Design review of the part built by this model. Coordinates are the model's own, in mm. A direction names the side the tool comes from. Coordinates: 2 decimals unless noted, no trailing zeros. Write each loop counter-clockwise with the first axis right and the second up, starting at its lowest first coordinate (ties: lowest second). Pieces come first, ordered by that corner, then holes. Notation, with made-up numbers: (54.5, 48.25) -> (66.5, 48.25) arc R12 cw to (66.5, 55.25) -> close; hole circle Ø11 at (42.5, 39). An arc over 180 degrees is marked (long way). Answer in a Markdown table with one row per item. Add a question column.
Item 1: Take a section at D-D, the plane x = -70.5. Write out the cut boundary in (y, z), and give its area (3 significant figures).
Item 2: Take a section at B-B, the plane z = -40. Write out the cut boundary in (x, y), and give its area (3 significant figures).
Item 3: For faces 1 (the face through (-39.44, 22.6, -15.77)), 2 (the face through (-40, -160, -40)), 3 (the face through (-32.68, -78.88, -41.63)), list the 3-axis set-ups (+Z, -Z, +X, -X, +Y, -Y) from which the entire face can be reached by the end or side of a thin tool; tool diameter is ignored.
Item 4: To check wall thickness, follow line 1 (Y direction, x = -27, z = -31); line 2 (Y direction, x = -51, z = -12.5); line 3 (Y direction, x = -41, z = -25). State the ranges of each line that lie inside material, in increasing order.
Item 5: Take a section at C-C, the plane x = -40. Write out the cut boundary in (y, z), and give its area (3 significant figures).
Item 6: Clearance check with flat-ended pins moving along their axes: P1, Ø10, axis at x = -30.5, y = -100.5, coming from the +Z side; P2, Ø10, axis at y = -92.5, z = -41, coming from the +X side; P3, Ø3, axis at y = -26.5, z = -36.5, coming from the -X side. State where each tip first meets the part, or that it passes through.
Item 7: Take a section at A-A, the plane y = -138.5. Write out the cut boundary in (x, z).
from build123d import *

# Parameters (mm, degrees)
SKETCH1_W           = 80
SKETCH1_H           = 48
BOSS_EXTRUDE1_DEPTH = 30
CUT_EXTRUDE1_DEPTH  = 99
CUT_EXTRUDE2_DEPTH  = 99
SKETCH4_R           = 7.5
BOSS_EXTRUDE2_DEPTH = 160


with BuildPart() as part:
    # Sketch1 → Boss-Extrude1 (new body)
    with BuildSketch(Plane(origin=(0, 0, 0), x_dir=(1, 0, 0), z_dir=(0, 1, 0))):
        with Locations((-40, 24)):
            Rectangle(SKETCH1_W, SKETCH1_H)
    extrude(amount=BOSS_EXTRUDE1_DEPTH)

    # Sketch2 → Cut-Extrude1 (cut, through all)
    with BuildSketch(Plane(origin=(0, 0, 0), x_dir=(0, 0, -1), z_dir=(1, 0, 0))):
        Polygon((0, 0), (15, 30), (0, 30), align=None)
        Polygon((48, 0), (33, 30), (48, 30), align=None)
    extrude(amount=-CUT_EXTRUDE1_DEPTH, mode=Mode.SUBTRACT)

    # Sketch3 → Cut-Extrude2 (cut, through all)
    with BuildSketch(Plane(origin=(0, 0, 0), x_dir=(0, 0, -1), z_dir=(1, 0, 0))):
        Polygon((19.472135955, 30), (11.972135955, 15), (36.027864045, 15), (28.527864045, 30), align=None)
    extrude(amount=-CUT_EXTRUDE2_DEPTH, mode=Mode.SUBTRACT)

    # Sketch4 → Boss-Extrude2 (add)
    with BuildSketch(Plane.XZ):
        with Locations(Location((-40, -20, 0), (0, 0, 270))):
            Circle(SKETCH4_R)
        with Locations(Location((-40, -40, 0), (0, 0, 90))):
            Circle(SKETCH4_R)
    extrude(amount=BOSS_EXTRUDE2_DEPTH)


solid = part.part
Answers:
| question | item | result |
|---|---|---|
| 1 | outline | (0, -48) -> (30, -33) -> (30, -28.53) -> (15, -36.03) -> (15, -11.97) -> (30, -19.47) -> (30, -15) -> (0, 0) -> close |
| 1 | area | 742 mm^2 |
| 2 | outline | (-80, 0) -> (-47.5, 0) -> (-47.5, -160) -> (-32.5, -160) -> (-32.5, 0) -> (0, 0) -> (0, 16) -> (-80, 16) -> close |
| 2 | area | 3,680 mm^2 |
| 3 | face 1 | +X, -X |
| 3 | face 2 | +Z, -Z, +X, -X, -Y |
| 3 | face 3 | -Y |
| 4 | line 1 | y = 0 to 15, 25.06 to 30 |
| 4 | line 2 | y = 0 to 15, 16.06 to 25 |
| 4 | line 3 | y = -160 to 15 |
| 5 | outline | (-160, -47.5) -> (0, -47.5) -> (0, -48) -> (30, -33) -> (30, -28.53) -> (15, -36.03) -> (15, -11.97) -> (30, -19.47) -> (30, -15) -> (0, 0) -> (0, -12.5) -> (-160, -12.5) -> (-160, -27.5) -> (0, -27.5) -> (0, -32.5) -> (-160, -32.5) -> close |
| 5 | area | 5,540 mm^2 |
| 6 | P1 | stops at z = -14 |
| 6 | P2 | stops at x = -32.5 |
| 6 | P3 | stops at x = -47.23 |
| 7 | outline | circle Ø15 at (-40, -40); circle Ø15 at (-40, -20) |
